Design review of the part shown in the three views and the two pictorial views. Dimensions are in mm from the part's minimum x, y and z. A direction names the side the tool comes from. Coordinates: 2 decimals unless noted, no trailing zeros. Write each loop counter-clockwise with the first axis right and the second up, starting at its lowest first coordinate (ties: lowest second). Pieces come first, ordered by that corner, then holes. Notation, with made-up numbers: M 36.25,79.25 L 55.25,79.25 A27 ccw 55.25,107.25 Z; hole C 7,-16.75 d10. An arc over 180 degrees is marked long. One line per question, with ' | ' between items.
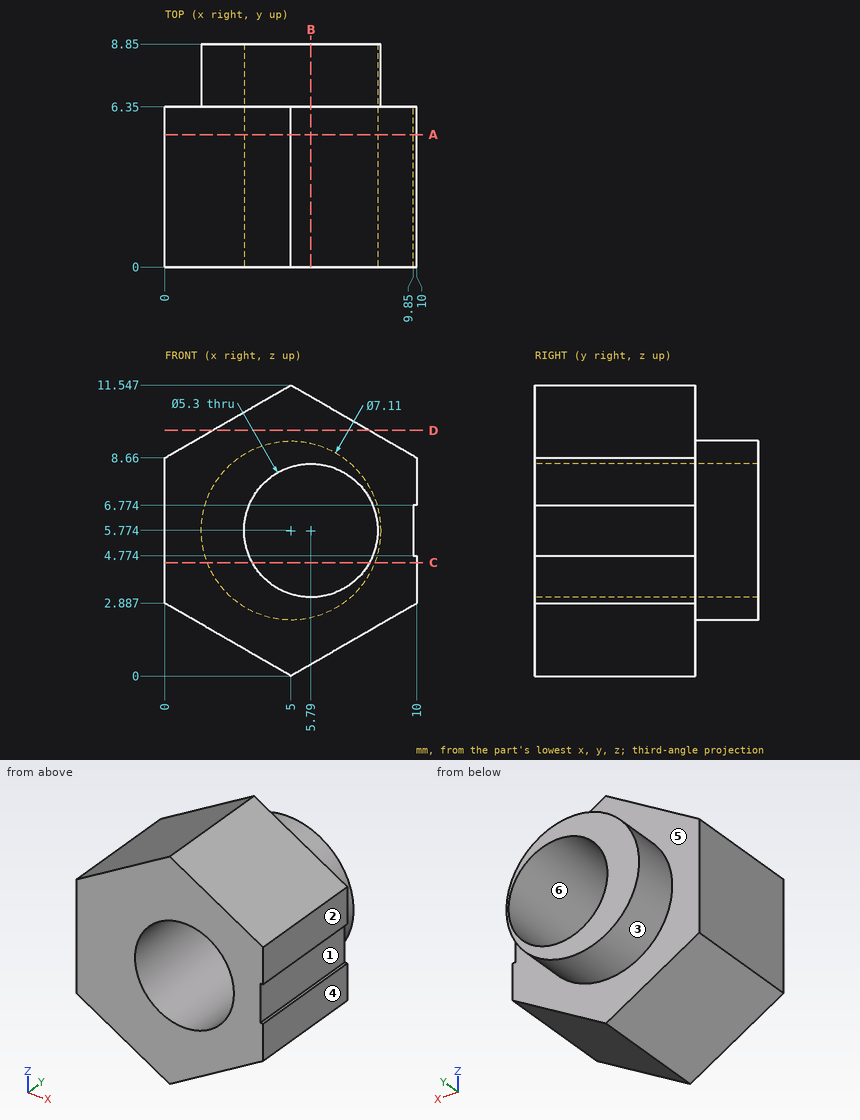
1. Machinability: for the marked faces 1, 2 and 3, which of the approach directions +Z, -Z, +X, -X, +Y, -Y give a long, thin tool a straight path to every point of the face, cutting with its end or side? Answer none if there is none.
Computed values:
face 1: +X, +Y, -Y | face 2: +Z, -Z, +X, +Y, -Y | face 3: +Y
2. Take a section at C-C on z = 4.5. State the section outline as (x, y) points.
Computed values:
outline: M 0,0 L 3.47,0 L 3.47,8.85 L 1.68,8.85 L 1.68,6.35 L 0,6.35 Z; M 8.11,0 L 10,0 L 10,6.35 L 8.32,6.35 L 8.32,8.85 L 8.11,8.85 Z
3. Clearance check with a flat-ended pin moving along its axis: P1, Ø0.6, axis at y = 2.5, z = 5.5, coming from the +X side. State where the tip first meets the part, or that it passes through.
Computed values:
P1: stops at x = 9.85
4. Take a section at B-B on x = 5.79. State the section outline as (y, z) points.
Computed values:
outline: M 0,0.46 L 6.35,0.46 L 6.35,2.31 L 8.85,2.31 L 8.85,3.12 L 0,3.12 Z; M 0,8.42 L 8.85,8.42 L 8.85,9.24 L 6.35,9.24 L 6.35,11.09 L 0,11.09 Z
5. Take a section at A-A on y = 5.25. State the section outline as (x, z) points.
Computed values:
outline: M 0,2.89 L 5,0 L 10,2.89 L 10,4.77 L 9.85,4.77 L 9.85,6.77 L 10,6.77 L 10,8.66 L 5,11.55 L 0,8.66 Z; hole C 5.79,5.77 d5.3
6. Draft analysis for pull direction X (two halves, no side actions). For the marked faces 4, 5 and 6, state which applies: pulls with the +X half, pulls with the -X half, needs draft (parallel to the pull), parting line crosses it, or undercut.
Computed values:
face 4: pulls with the +X half | face 5: needs draft | face 6: undercut
7. Take a section at D-D on z = 9.75. State the section outline as (x, y) points.
Computed values:
outline: M 1.89,0 L 8.11,0 L 8.11,6.35 L 1.89,6.35 Z
8. For line 1 along X through (y, z) = (1, 4.5) (1 decimal); line 2 along Z through (x, y) = (5.79, 6) (1 decimal); line 3 along Z through (x, y) = (5.75, 1.5) (1 decimal), list the stretches that pass through material, from the lowest coordinate up.
Computed values:
line 1: x = 0 to 3.5, 8.1 to 10 | line 2: z = 0.5 to 3.1, 8.4 to 11.1 | line 3: z = 0.4 to 3.1, 8.4 to 11.1
